Could you check a few things on this model? Use its own coordinates, in mm. A direction names the side the tool comes from. Coordinates: 2 decimals unless noted, no trailing zeros. Write each loop counter-clockwise with the first axis right and the second up, starting at its lowest first coordinate (ties: lowest second). Pieces come first, ordered by that corner, then holes.
Item 1: Which directions (+Z, -Z, +X, -X, +Y, -Y) give clear straight access to the entire face, cutting with the end or side of a thin tool? Please do faces 1 (the flat face through (5, 56.15, 3)), 2 (the flat face through (38, 37.95, -9)), 3 (the flat face through (47, 36, 9.77)).
Item 2: For P1, Ø8, axis at x = 52, y = 49, coming from the +Z side; P2, Ø5, axis at y = -4, z = 2.5, coming from the +X side; P3, Ø3, axis at x = 55.5, y = 31.5, coming from the -Z side; P4, Ø6, axis at y = -8, z = -7, coming from the -X side, each with a flat end and sliding along its axis, tell me the tip position at first contact or that it passes through.
Item 3: I want a section at B-B on y = 43. Please give me the cut outline in (x, z).
Item 4: Thinking about a two-plate mould opening in Z: for faces 4 (the flat face through (80, 20, -6.95)), 5 (the flat face through (63, -10, 16.7)), 6 (the cylindrical face through (2.715, 39.668, -3.611)), 7 (the flat face through (46, 36, 0)), which applies, +Z half, -Z half, draft (parallel to the pull), parting line (faces both ways), or undercut?
Item 5: If I drill on probe 1 along Z at (x, y) = (50, 19.5); probe 2 along Y at (x, z) = (34.5, -5.5); probe 3 along X at (y, z) = (38, -6.5), over which ranges is the centre line in solid material (lowest first)?
from build123d import *
from build123d.topology import SkipClean

# Parameters (mm, degrees)
SKETCH1_W            = 93.06
SKETCH1_H            = 70.1
SKETCH1_R            = 1.525
BOSS_EXTRUDE1_DEPTH  = 1.57
SKETCH2_W            = 78.1
SKETCH2_H            = 51
BOSS_EXTRUDE2_DEPTH  = 8.4
CUT_EXTRUDE1_DEPTH   = 0.2
SKETCH4_W            = 5.7
SKETCH4_H            = 42.1
BOSS_EXTRUDE3_DEPTH  = 3.3
SKETCH6_W            = 93.06
SKETCH6_H            = 60.05
BOSS_EXTRUDE4_DEPTH  = 1.6
SKETCH7_R            = 2
CUT_EXTRUDE2_DEPTH   = 1.6
BOSS_EXTRUDE5_REACH  = 118.934
SKETCH8_W            = 73.06
SKETCH8_H            = 2
SKETCH9_W            = 20.3
SKETCH9_H            = 8.75
SKETCH9_W_2          = 19.3
SKETCH9_H_2          = 7.75
BOSS_EXTRUDE6_DEPTH  = 9
BOSS_EXTRUDE7_DEPTH  = 3.05
CUT_EXTRUDE3_REACH   = 119.276
SKETCH11_W           = 2.05
SKETCH11_H           = 25.35
BOSS_EXTRUDE8_DEPTH  = 3.05
BOSS_EXTRUDE9_DEPTH  = 3.5
SKETCH15_R           = 1.75
BOSS_EXTRUDE10_DEPTH = 1.6
BOSS_EXTRUDE11_DEPTH = 5.8
SKETCH17_R           = 3.425
BOSS_EXTRUDE12_DEPTH = 4.7
BOSS_EXTRUDE13_DEPTH = 9
SKETCH19_R           = 0.6
BOSS_EXTRUDE14_DEPTH = 0.4
SKETCH21_R           = 5.9
BOSS_EXTRUDE15_DEPTH = 9.5
SKETCH22_R           = 1.2
CUT_EXTRUDE4_DEPTH   = 2
SKETCH23_R           = 3
BOSS_EXTRUDE16_DEPTH = 2


with BuildPart() as part:
    # Sketch1 → Boss-Extrude1 (new body)
    with BuildSketch(Plane.XY):
        with Locations((46.53, 35.05)):
            Rectangle(SKETCH1_W, SKETCH1_H)
        with Locations((2.455, 67.565)):
            Circle(SKETCH1_R, mode=Mode.SUBTRACT)
        with Locations((90.605, 67.565)):
            Circle(SKETCH1_R, mode=Mode.SUBTRACT)
        with Locations((90.605, 2.535)):
            Circle(SKETCH1_R, mode=Mode.SUBTRACT)
        with Locations((2.455, 2.535)):
            Circle(SKETCH1_R, mode=Mode.SUBTRACT)
    extrude(amount=BOSS_EXTRUDE1_DEPTH)

    # Sketch2 → Boss-Extrude2 (add)
    with BuildSketch(Plane.XY.offset(1.57)):
        with Locations((46.66, 35.25)):
            Rectangle(SKETCH2_W, SKETCH2_H)
    extrude(amount=BOSS_EXTRUDE2_DEPTH)

    # Sketch3 → Cut-Extrude1 (cut)
    with BuildSketch(Plane.XY.offset(9.97)):
        with BuildLine():
            Line((11.61, 55.25), (81.71, 55.25))
            ThreePointArc((81.71, 55.25), (82.417106781, 54.957106781), (82.71, 54.25))
            Line((82.71, 54.25), (82.71, 16.25))
            ThreePointArc((82.71, 16.25), (82.417106781, 15.542893219), (81.71, 15.25))
            Line((81.71, 15.25), (11.61, 15.25))
            ThreePointArc((11.61, 15.25), (10.902893219, 15.542893219), (10.61, 16.25))
            Line((10.61, 16.25), (10.61, 54.25))
            ThreePointArc((10.61, 54.25), (10.902893219, 54.957106781), (11.61, 55.25))
        make_face()
    extrude(amount=-CUT_EXTRUDE1_DEPTH, mode=Mode.SUBTRACT)

    # Sketch4 → Boss-Extrude3 (add)
    with BuildSketch(Plane.XY.offset(1.57)):
        with Locations((4.76, 35.1)):
            Rectangle(SKETCH4_W, SKETCH4_H)
    extrude(amount=BOSS_EXTRUDE3_DEPTH)


with BuildPart() as body_2:
    # Sketch6 → Boss-Extrude4 (new body)
    with BuildSketch(Plane(origin=(0, 0, -2.8), x_dir=(-1, 0, 0), z_dir=(0, 0, -1))):
        with Locations((-46.53, 10.075)):
            Rectangle(SKETCH6_W, SKETCH6_H)
    extrude(amount=BOSS_EXTRUDE4_DEPTH)

    # Sketch7 → Cut-Extrude2 (cut)
    with BuildSketch(Plane(origin=(0, 0, -4.4), x_dir=(-1, 0, 0), z_dir=(0, 0, -1))):
        with Locations((-90.605, 37.685)):
            Circle(SKETCH7_R)
        with Locations((-90.605, -17.565)):
            Circle(SKETCH7_R)
        with Locations((-2.455, -17.565)):
            Circle(SKETCH7_R)
        with Locations((-2.455, 37.685)):
            Circle(SKETCH7_R)
        with Locations((-90.605, 2.535)):
            Circle(SKETCH7_R)
        with Locations((-2.455, 2.535)):
            Circle(SKETCH7_R)
    extrude(amount=-CUT_EXTRUDE2_DEPTH, mode=Mode.SUBTRACT)

    # Sketch8 → Boss-Extrude5 (add, up to next)
    with BuildSketch(Plane(origin=(0, 0, 0), x_dir=(-1, 0, 0), z_dir=(0, 0, -1)), mode=Mode.PRIVATE) as boss_extrude5_sk1:
        with Locations((-46.53, 11)):
            Rectangle(SKETCH8_W, SKETCH8_H)
    boss_extrude5_tool1 = extrude(boss_extrude5_sk1.sketch, amount=BOSS_EXTRUDE5_REACH, mode=Mode.PRIVATE) - body_2.part
    # Sketch8 → Boss-Extrude5 (add, up to next)
    with BuildSketch(Plane(origin=(0, 0, 0), x_dir=(-1, 0, 0), z_dir=(0, 0, -1)), mode=Mode.PRIVATE) as boss_extrude5_sk2:
        with Locations((-46.53, 29.1)):
            Rectangle(SKETCH8_W, SKETCH8_H)
    boss_extrude5_tool2 = extrude(boss_extrude5_sk2.sketch, amount=BOSS_EXTRUDE5_REACH, mode=Mode.PRIVATE) - body_2.part

    add(part.part)  # Boss-Extrude5 merges part
    add(boss_extrude5_tool1.solids().sort_by_distance((46.53, 11, 0))[0])
    add(boss_extrude5_tool2.solids().sort_by_distance((46.53, 29.1, 0))[0])

    # Sketch9 → Boss-Extrude6 (add)
    # profile 1 of 2: a face of its own
    with BuildSketch(Plane(origin=(0, 0, -4.4), x_dir=(-1, 0, 0), z_dir=(0, 0, -1))):
        with Locations((-37.65, 34.075)):
            Rectangle(SKETCH9_W, SKETCH9_H)
        with Locations((-37.65, 34.075)):
            Rectangle(SKETCH9_W_2, SKETCH9_H_2, mode=Mode.SUBTRACT)
    # profile 2 of 2: a face of its own
    with BuildSketch(Plane(origin=(0, 0, -4.4), x_dir=(-1, 0, 0), z_dir=(0, 0, -1))):
        with Locations((-16.65, 34.075)):
            Rectangle(SKETCH9_W, SKETCH9_H)
        with Locations((-16.65, 34.075)):
            Rectangle(SKETCH9_W_2, SKETCH9_H_2, mode=Mode.SUBTRACT)
    extrude(amount=BOSS_EXTRUDE6_DEPTH)

    # Sketch10 → Boss-Extrude7 (add)
    with BuildSketch(Plane(origin=(0, 0, -4.4), x_dir=(-1, 0, 0), z_dir=(0, 0, -1))):
        Polygon((-93.06, 33.7), (-66.46, 33.7), (-66.46, 9.35), (-71.86, 9.35), (-75.06, 7.35), (-93.06, 7.35), align=None)
    extrude(amount=BOSS_EXTRUDE7_DEPTH)

    # Sketch11 → Cut-Extrude3 (cut, up to next)
    with BuildSketch(Plane(origin=(93.06, 0, 0), x_dir=(0, 0, -1), z_dir=(1, 0, 0)), mode=Mode.PRIVATE) as cut_extrude3_sk1:
        with Locations((5.925, 20.525)):
            Rectangle(SKETCH11_W, SKETCH11_H)
    cut_extrude3_tool1 = extrude(cut_extrude3_sk1.sketch, amount=-CUT_EXTRUDE3_REACH, mode=Mode.PRIVATE) & body_2.part
    add(cut_extrude3_tool1.solids().sort_by_distance((93.06, 20.525, -5.925))[0], mode=Mode.SUBTRACT)

    # Sketch12 → Boss-Extrude8 (add)
    with BuildSketch(Plane(origin=(0, 0, -7.45), x_dir=(-1, 0, 0), z_dir=(0, 0, -1))):
        Polygon((-75.06, 7.35), (-71.86, 9.35), (-66.46, 9.35), (-66.46, 33.7), (-66.96, 33.7), (-66.96, 9.85), (-72.003398113, 9.85), (-75.203398113, 7.85), (-77.778406171, 7.85), (-77.778406171, 7.35), align=None)
    extrude(amount=-BOSS_EXTRUDE8_DEPTH)

    # Sketch14 → Boss-Extrude9 (add)
    with BuildSketch(Plane.XY.offset(-2.8)):
        with BuildLine():
            Line((78.66, -9.65), (84.26, -9.65))
            ThreePointArc((84.26, -9.65), (84.401421356, -9.708578644), (84.46, -9.85))
            Line((84.46, -9.85), (84.46, -15.45))
            ThreePointArc((84.46, -15.45), (84.401421356, -15.591421356), (84.26, -15.65))
            Line((84.26, -15.65), (78.66, -15.65))
            ThreePointArc((78.66, -15.65), (78.518578644, -15.591421356), (78.46, -15.45))
            Line((78.46, -15.45), (78.46, -9.85))
            ThreePointArc((78.46, -9.85), (78.518578644, -9.708578644), (78.66, -9.65))
        make_face()
        with BuildLine():
            Line((46.51, -9.85), (52.11, -9.85))
            ThreePointArc((52.11, -9.85), (52.251421356, -9.908578644), (52.31, -10.05))
            Line((52.31, -10.05), (52.31, -15.65))
            ThreePointArc((52.31, -15.65), (52.251421356, -15.791421356), (52.11, -15.85))
            Line((52.11, -15.85), (46.51, -15.85))
            ThreePointArc((46.51, -15.85), (46.368578644, -15.791421356), (46.31, -15.65))
            Line((46.31, -15.65), (46.31, -10.05))
            ThreePointArc((46.31, -10.05), (46.368578644, -9.908578644), (46.51, -9.85))
        make_face()
    extrude(amount=BOSS_EXTRUDE9_DEPTH)

    # Sketch15 → Boss-Extrude10 (add)
    with BuildSketch(Plane.XY.offset(0.7)):
        with Locations((49.31, -12.85)):
            Circle(SKETCH15_R)
        with Locations((81.46, -12.65)):
            Circle(SKETCH15_R)
    extrude(amount=BOSS_EXTRUDE10_DEPTH)

    # Sketch16 → Boss-Extrude11 (add)
    with BuildSketch(Plane.XY.offset(-2.8)):
        with BuildLine():
            Line((57.51, -3.05), (69.16, -3.05))
            ThreePointArc((69.16, -3.05), (69.513553391, -3.196446609), (69.66, -3.55))
            Line((69.66, -3.55), (69.66, -15.85))
            ThreePointArc((69.66, -15.85), (69.513553391, -16.203553391), (69.16, -16.35))
            Line((69.16, -16.35), (57.51, -16.35))
            ThreePointArc((57.51, -16.35), (57.156446609, -16.203553391), (57.01, -15.85))
            Line((57.01, -15.85), (57.01, -3.55))
            ThreePointArc((57.01, -3.55), (57.156446609, -3.196446609), (57.51, -3.05))
        make_face()
    extrude(amount=BOSS_EXTRUDE11_DEPTH)

    # Sketch17 → Boss-Extrude12 (add)
    with BuildSketch(Plane.XY.offset(3)):
        with Locations((63.335, -9.7)):
            Circle(SKETCH17_R)
    extrude(amount=BOSS_EXTRUDE12_DEPTH)

    # Sketch18 → Boss-Extrude13 (add)
    with BuildSketch(Plane.XY.offset(7.7)):
        with BuildLine():
            Line((60.708690803, -8.25), (65.961309197, -8.25))
            ThreePointArc((65.961309197, -8.25), (63.335, -12.7), (60.708690803, -8.25))
        make_face()
    extrude(amount=BOSS_EXTRUDE13_DEPTH)

    # Sketch19 → Boss-Extrude14 (add)
    with BuildSketch(Plane.XY.offset(0.7)):
        with Locations((79.31, -10.5)):
            Circle(SKETCH19_R)
        with Locations((83.61, -10.5)):
            Circle(SKETCH19_R)
        with Locations((83.61, -14.8)):
            Circle(SKETCH19_R)
        with Locations((79.31, -14.8)):
            Circle(SKETCH19_R)
        with Locations((47.16, -10.7)):
            Circle(SKETCH19_R)
        with Locations((51.46, -10.7)):
            Circle(SKETCH19_R)
        with Locations((51.46, -15)):
            Circle(SKETCH19_R)
        with Locations((47.16, -15)):
            Circle(SKETCH19_R)
    extrude(amount=BOSS_EXTRUDE14_DEPTH)

    # Sketch21 → Boss-Extrude15 (add)
    with BuildSketch(Plane.XY.offset(-2.8)):
        with Locations(Location((28, -10.85, 0), (0, 0, 180))):
            Circle(SKETCH21_R)
    extrude(amount=BOSS_EXTRUDE15_DEPTH)

    # Sketch22 → Cut-Extrude4 (cut)
    with BuildSketch(Plane.XY.offset(6.7)):
        with Locations((28, -10.85)):
            Circle(SKETCH22_R)
    extrude(amount=-CUT_EXTRUDE4_DEPTH, mode=Mode.SUBTRACT)

    # Sketch23 → Boss-Extrude16 (add)
    with SkipClean():  # the faces are left unmerged after this step: merging them gives an invalid solid
        with BuildSketch(Plane.XY.offset(7.7)):
            with Locations(Location((63.335, -9.7, 0), (0, 0, 151.09666546))):
                Circle(SKETCH23_R)
        extrude(amount=BOSS_EXTRUDE16_DEPTH)


solid = body_2.part
Response values:
1. face 1: +Z, -X, +Y
1. face 2: -Z
1. face 3: +Z
2. P1: stops at z = 9.77
2. P2: stops at x = 69.66
2. P3: stops at z = -4.4
2. P4: stops at x = 0
3. outline: (0, 0) - (93.06, 0) - (93.06, 1.57) - (85.71, 1.57) - (85.71, 9.97) - (82.71, 9.97) - (82.71, 9.77) - (10.61, 9.77) - (10.61, 9.97) - (7.61, 9.97) - (7.61, 4.87) - (1.91, 4.87) - (1.91, 1.57) - (0, 1.57) - close
4. face 4: undercut
4. face 5: +Z half
4. face 6: draft
4. face 7: undercut
5. probe 1: z = -4.4 to -2.8, 0 to 9.77
5. probe 2: y = 29.7 to 30.2, 37.95 to 38.45
5. probe 3: x = 6.5 to 26.8, 27.5 to 47.8
